```python
from build123d import *

# Parameters (mm, degrees)
SKETCH1_R           = 95.25
BOSS_EXTRUDE1_DEPTH = 12.7
SKETCH2_R           = 3.175
CUT_EXTRUDE1_DEPTH  = 26.4
CIRPATTERN1_COUNT   = 3
SKETCH3_R           = 2.8448
CUT_EXTRUDE2_DEPTH  = 12.7
CIRPATTERN2_COUNT   = 3


with BuildPart() as part:
    # Sketch1 → Boss-Extrude1 (new body, symmetric)
    with BuildSketch(Plane(origin=(0, 0, 0), x_dir=(1, 0, 0), z_dir=(0, 1, 0))):
        Circle(SKETCH1_R)
    extrude(amount=BOSS_EXTRUDE1_DEPTH, both=True)

    # Sketch2 → Cut-Extrude1 (cut, through all)
    with BuildSketch(Plane(origin=(0, 12.7, 0), x_dir=(1, 0, 0), z_dir=(0, 1, 0))):
        with Locations((0, 89.535)):
            Circle(SKETCH2_R)
    cut_extrude1 = extrude(amount=-CUT_EXTRUDE1_DEPTH, mode=Mode.SUBTRACT)

    # CirPattern1: Cut-Extrude1 ×3 about axis
    cirpattern1_axis = Axis((0, 0, 0), (0, 1, 0))
    for i in range(1, CIRPATTERN1_COUNT):
        add(cut_extrude1.rotate(cirpattern1_axis, i * 360 / CIRPATTERN1_COUNT), mode=Mode.SUBTRACT)

    # Sketch3 → Cut-Extrude2 (cut)
    with BuildSketch(Plane(origin=(0, -12.7, 0), x_dir=(-1, 0, 0), z_dir=(0, -1, 0))):
        with Locations((-77.539584528, 44.7675)):
            Circle(SKETCH3_R)
    cut_extrude2 = extrude(amount=-CUT_EXTRUDE2_DEPTH, mode=Mode.SUBTRACT)

    # CirPattern2: Cut-Extrude2 ×3 about axis
    cirpattern2_axis = Axis((0, 0, 0), (0, 1, 0))
    for i in range(1, CIRPATTERN2_COUNT):
        add(cut_extrude2.rotate(cirpattern2_axis, i * 360 / CIRPATTERN2_COUNT), mode=Mode.SUBTRACT)


solid = part.part
```
Here's how the part is built. I have some questions about the finished solid (model axes, mm). A direction names the side the tool comes from. Give positions to 0.01 mm unless a question says otherwise; leave off trailing zeros. Loops run counter-clockwise (first coordinate to the right, second up) from the corner with the lowest first, then second, coordinate; pieces in that order, holes last. Notation, with made-up numbers: M 38,-21 L 59,-21 A35 ccw 59,11 Z; hole C -36.5,-4 d1. An arc over 180 degrees is marked long. Put each result on its own line as item: value. Start each with the question number.
(1) If we mould it in two halves opening along X, with no side actions, what happens to faces 1 (the cylindrical face through (0.62, -6.44, 92.31)), 2 (the flat face through (-1, 12.7, -1)), 3 (the cylindrical face through (-75.587, 0.178, 57.958))? For each: +X half, -X half, draft (parallel to the pull), parting line (faces both ways), or undercut.
(2) For faces 4 (the flat face through (-1, -12.7, -1)), 5 (the flat face through (-78, 0, -45)), which set-ups out of +Z, -Z, +X, -X, +Y, -Y let a thin tool reach every point of the face, with its end or its side?
(3) I want a section at A-A on y = -6.75. State how many separate pieces and enclosed holes the cut face has, then the cut area to 3 significant figures.
(4) Will these pins go through, and if not, where does the flat tip stop? pin 1 Ø1 at (x, y) = (-55, -2) entering from -Z; pin 2 Ø6.5 at (x, z) = (77.54, -44.77) entering from -Y; pin 3 Ø12 at (y, z) = (-7, -50) entering from +X; pin 4 Ø5 at (x, y) = (19, 2) entering from -Z.
(5) I want a section at C-C on x = 47.5. Please give me the cut outline in (y, z).
(6) I want a section at B-B on z = 19. Please give me the cut outline in (x, y), then the cut area to 3 significant figures.
(7) I need wall thicknesses on line 1 along Z through (x, y) = (0, -3.25); line 2 along X through (y, z) = (-7.5, 42); line 3 along Z through (x, y) = (1.5, -6.5). Which ranges of each line are inside material? Lowest first, please. Write a range as [from, to].
Answer block:
1. face 1: undercut
1. face 2: draft
1. face 3: parting line
2. face 4: +Z, -Z, +X, -X, -Y
2. face 5: -Y
3. separate pieces: 1
3. enclosed holes: 6
3. area: 28,300 mm^2
4. pin 1: z = -78.12
4. pin 2: y = -12.7
4. pin 3: x = 84.48
4. pin 4: z = -93.81
5. outline: M -12.7,-82.56 L 12.7,-82.56 L 12.7,82.56 L -12.7,82.56 Z
6. outline: M -93.34,-12.7 L 93.34,-12.7 L 93.34,12.7 L -93.34,12.7 Z
6. area: 4,740 mm^2
7. line 1: [-95.25, -92.71], [-86.36, 86.69], [92.38, 95.25]
7. line 2: [-85.49, -79.1], [-75.98, 75.98], [79.1, 85.49]
7. line 3: [-95.24, -92.33], [-86.74, 87.12], [91.95, 95.24]
